Input: part model. Units: mm. Frame: model coordinates. Coordinates: 2 decimals unless noted, no trailing zeros. Loops run counter-clockwise (first coordinate to the right, second up) from the corner with the lowest first, then second, coordinate; pieces in that order, holes last. Notation, with made-up numbers: (56, 56.25) -> (67, 56.25) arc R24 ccw to (67, 83.25) -> close; hole circle Ø10 at (35, -24). An arc over 180 degrees is marked (long way). Answer as a JSON object with one key per item and string values.
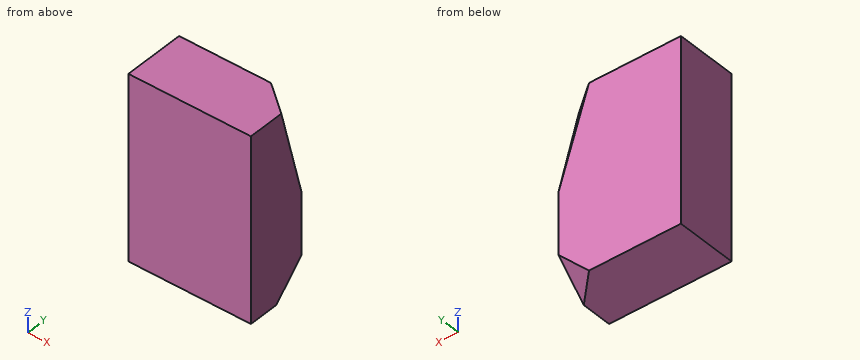
from build123d import *

# Parameters (mm, degrees)
SKETCH1_W           = 101.6
SKETCH1_H           = 152.4
BOSS_EXTRUDE2_DEPTH = 50.8
CUT_EXTRUDE1_DEPTH  = 141.672729153
CUT_EXTRUDE2_DEPTH  = 171.388379885


with BuildPart() as part:
    # Sketch1 → Boss-Extrude2 (new body)
    with BuildSketch(Plane(origin=(0, 0, 0), x_dir=(1, 0, 0), z_dir=(0, 1, 0))):
        Rectangle(SKETCH1_W, SKETCH1_H)
    extrude(amount=BOSS_EXTRUDE2_DEPTH)

    # Sketch5 → Cut-Extrude1 (cut, through all)
    with BuildSketch(Plane(origin=(42.751168831, 53.438961039, 14.25038961), x_dir=(0.7911852033335972, -0.5909267078840152, -0.15758045543573734), z_dir=(0.6115766297251511, 0.764470787156438, 0.20385887657505006))):
        Polygon((-21.9306033, -60.537839749), (10.173131569, 13.089262648), (10.173131569, -65.773544809), align=None)
    extrude(amount=CUT_EXTRUDE1_DEPTH, mode=Mode.SUBTRACT)

    # Sketch7 → Cut-Extrude2 (cut, through all)
    with BuildSketch(Plane(origin=(50.8, 50.8, -50.8), x_dir=(0.8164965809277263, -0.40824829046386296, 0.40824829046386296), z_dir=(-0.5773502691896256, -0.5773502691896258, 0.5773502691896258))):
        Polygon((0, 0), (0, -35.921024484), (-31.108519733, -17.960512242), align=None)
    extrude(amount=-CUT_EXTRUDE2_DEPTH, mode=Mode.SUBTRACT)


solid = part.part
1. Section query A-A (x = 40). Return loops of the section in (y, z), plus the area to 3 significant figures.
Reply:
{"outline": "(0, -76.2) -> (36.2, -76.2) -> (50.8, -61.6) -> (50.8, 32.4) -> (39.12, 76.2) -> (0, 76.2) -> close", "area": "7,380 mm2"}
2. Line query: line 1 along X through (y, z) = (39.5, 61); line 2 along X through (y, z) = (43.5, 41). Output: solid intervals per line, ascending.
Reply:
{"line 1": "x = -50.8 to 44.59", "line 2": "x = -50.8 to 46.26"}
3. Section query C-C (y = 40.5). Return loops of the section in (x, z) (3 decimals).
Reply:
{"outline": "(-50.8, -76.2) -> (35.7, -76.2) -> (50.8, -61.1) -> (50.8, 38.625) -> (38.275, 76.2) -> (-50.8, 76.2) -> close"}
4. Section query B-B (z = 50.5). Return loops of the section in (x, y).
Reply:
{"outline": "(-50.8, 0) -> (50.8, 0) -> (50.8, 37.33) -> (33.97, 50.8) -> (-50.8, 50.8) -> close"}
